```python
from build123d import *

# Parameters (mm, degrees)
CROQUIS1_W              = 8
CROQUIS1_H              = 28.768453788
SALIENTE_EXTRUIR1_DEPTH = 50
CORTAR_EXTRUIR1_REACH   = 10
CROQUIS3_R              = 1.6
CROQUIS4_R              = 1.95
CORTAR_EXTRUIR2_DEPTH   = 22


with BuildPart() as part:
    # Croquis1 → Saliente-Extruir1 (new body)
    with BuildSketch(Plane.XY):
        with Locations((90, 9.384226894)):
            Rectangle(CROQUIS1_W, CROQUIS1_H)
    extrude(amount=SALIENTE_EXTRUIR1_DEPTH)

    # Croquis3 → Cortar-Extruir1 (cut, up to next)
    with BuildSketch(Plane(origin=(86, 0, 0), x_dir=(0, 0, -1), z_dir=(1, 0, 0)), mode=Mode.PRIVATE) as cortar_extruir1_sk1:
        with Locations((-43.227046774, 1.729227937)):
            Circle(CROQUIS3_R)
    cortar_extruir1_tool1 = extrude(cortar_extruir1_sk1.sketch, amount=CORTAR_EXTRUIR1_REACH, mode=Mode.PRIVATE) & part.part
    add(cortar_extruir1_tool1.solids().sort_by_distance((86, 1.729228, 43.227047))[0], mode=Mode.SUBTRACT)
    # Croquis3 → Cortar-Extruir1 (cut, up to next)
    with BuildSketch(Plane(origin=(86, 0, 0), x_dir=(0, 0, -1), z_dir=(1, 0, 0)), mode=Mode.PRIVATE) as cortar_extruir1_sk2:
        with Locations((-27.863523387, 10)):
            Circle(CROQUIS3_R)
    cortar_extruir1_tool2 = extrude(cortar_extruir1_sk2.sketch, amount=CORTAR_EXTRUIR1_REACH, mode=Mode.PRIVATE) & part.part
    add(cortar_extruir1_tool2.solids().sort_by_distance((86, 10, 27.863523))[0], mode=Mode.SUBTRACT)
    # Croquis3 → Cortar-Extruir1 (cut, up to next)
    with BuildSketch(Plane(origin=(86, 0, 0), x_dir=(0, 0, -1), z_dir=(1, 0, 0)), mode=Mode.PRIVATE) as cortar_extruir1_sk3:
        with Locations((-43.227046774, 18.270772063)):
            Circle(CROQUIS3_R)
    cortar_extruir1_tool3 = extrude(cortar_extruir1_sk3.sketch, amount=CORTAR_EXTRUIR1_REACH, mode=Mode.PRIVATE) & part.part
    add(cortar_extruir1_tool3.solids().sort_by_distance((86, 18.270772, 43.227047))[0], mode=Mode.SUBTRACT)

    # Croquis4 → Cortar-Extruir2 (cut)
    with BuildSketch(Plane(origin=(0, 0, 0), x_dir=(-1, 0, 0), z_dir=(0, 0, -1))):
        with Locations((-90.073577236, 1)):
            Circle(CROQUIS4_R)
        with Locations((-90, 9.384226894)):
            Circle(CROQUIS4_R)
        with Locations((-90, 17.768453788)):
            Circle(CROQUIS4_R)
    extrude(amount=-CORTAR_EXTRUIR2_DEPTH, mode=Mode.SUBTRACT)


solid = part.part
```
Check sheet for the modelled part. Datum: model origin and axes. Units: mm. A direction names the side the tool comes from. Give positions to 0.01 mm unless a question says otherwise; leave off trailing zeros. Write each loop counter-clockwise with the first axis right and the second up, starting at its lowest first coordinate (ties: lowest second). Pieces come first, ordered by that corner, then holes. Notation, with made-up numbers: (-38.5, 17) -> (13.5, 17) arc R15 ccw to (13.5, 42) -> close; hole circle Ø6 at (85.25, 1.5). An arc over 180 degrees is marked (long way). Use CSV: the item, a comma, the result in double quotes. Start each with the question number.
Q1. Depth check by flat-ended pin: P1, Ø3, axis at x = 89, y = 0.5, coming from the -Z side; P2, Ø3, axis at y = 18.27, z = 43.23, coming from the +X side; P3, Ø1.9, axis at x = 90, y = 18, coming from the -Z side. Enter the tip coordinate at first touch or a pass-through.
Q2. Cross-section at D-D on y = 1. Enter the section's corners in (x, z), and give its area (3 significant figures).
Q3. Cross-section at C-C on x = 87. Enter the section's corners in (y, z).
Q4. Cross-section at B-B on y = 10. Enter the section's corners in (x, z).
Q5. Release check for a two-part mould opening along Z. For faces 1 (the flat face through (86, 9, 25)), 2 (the flat face through (90, 18, 22)), 3 (the cylindrical face through (89.944, 18.341, 44.825)) record: +Z half, -Z half, draft (parallel to the pull), parting line (faces both ways), or undercut.
Q6. Tool access check on faces 4 (the flat face through (90, 10, 50)), 5 (the flat face through (90, 9, 22)). Record the directions out of +Z, -Z, +X, -X, +Y, -Y that give a thin tool (end or side, any length) a straight path to the whole face; none if there is none.
Q7. Cross-section at A-A on x = 90. Enter the section's corners in (y, z).
Q8. Scan lines: line 1 along Y through (x, z) = (90, 15.75); line 2 along Z through (x, y) = (88, 1.75); line 3 along Y through (x, z) = (88.5, 17). Record each from-to range of solid material in increasing order.
Working result:
1,P1,"stops at z = 0"
1,P2,"passes through"
1,P3,"stops at z = 22"
2,outline,"(86, 0) -> (88.12, 0) -> (88.12, 22) -> (92.02, 22) -> (92.02, 0) -> (94, 0) -> (94, 41.8) -> (86, 41.8) -> close; (86, 44.65) -> (94, 44.65) -> (94, 50) -> (86, 50) -> close"
2,area,"291 mm^2"
3,outline,"(-5, 0) -> (23.77, 0) -> (23.77, 50) -> (-5, 50) -> close; hole circle Ø3.2 at (1.73, 43.23); hole circle Ø3.2 at (10, 27.86); hole circle Ø3.2 at (18.27, 43.23)"
4,outline,"(86, 0) -> (88.15, 0) -> (88.15, 22) -> (91.85, 22) -> (91.85, 0) -> (94, 0) -> (94, 26.26) -> (86, 26.26) -> close; (86, 29.46) -> (94, 29.46) -> (94, 50) -> (86, 50) -> close"
5,face 1,"draft"
5,face 2,"-Z half"
5,face 3,"undercut"
6,face 4,"+Z, +X, -X, +Y, -Y"
6,face 5,"-Z"
7,outline,"(-5, 0) -> (-0.95, 0) -> (-0.95, 22) -> (2.95, 22) -> (2.95, 0) -> (7.43, 0) -> (7.43, 22) -> (11.33, 22) -> (11.33, 0) -> (15.82, 0) -> (15.82, 22) -> (19.72, 22) -> (19.72, 0) -> (23.77, 0) -> (23.77, 50) -> (-5, 50) -> close; hole circle Ø3.2 at (1.73, 43.23); hole circle Ø3.2 at (10, 27.86); hole circle Ø3.2 at (18.27, 43.23)"
8,line 1,"y = -5 to -0.95, 2.95 to 7.43, 11.33 to 15.82, 19.72 to 23.77"
8,line 2,"z = 0 to 41.63, 44.83 to 50"
8,line 3,"y = -5 to -0.15, 2.15 to 8.14, 10.63 to 16.52, 19.01 to 23.77"
